```python
from build123d import *

# Parameters (mm, degrees)
BOSS_EXTRUDE1_DEPTH = 17
SKETCH2_R           = 3.9
CUT_EXTRUDE1_DEPTH  = 7.9
CUT_EXTRUDE2_START  = -7.9
SKETCH3_R           = 3.9
CUT_EXTRUDE2_DEPTH  = 7.9
SKETCH4_R           = 2.7
CUT_EXTRUDE3_DEPTH  = 1.2
SHELL1_DEPTH        = 15.8
SKETCH8_R           = 0.5
CUT_EXTRUDE4_DEPTH  = 17


# Read off the part's stored shape, not the designer's step: Shell1
with BuildPart() as part:
    # Sketch1 → Boss-Extrude1 (new body)
    with BuildSketch(Plane(origin=(0, 0, 0), x_dir=(1, 0, 0), z_dir=(0, 1, 0))):
        with BuildLine():
            Line((-9.1, 2.7), (-9.1, -2.7))
            add(Edge.make_bspline(
                [(-9.1, -2.7), (0, -7.5), (9.1, -2.7)],
                knots=[0, 0, 0, 1, 1, 1], degree=2))
            Line((9.1, -2.7), (9.1, 2.7))
            add(Edge.make_bspline(
                [(-9.1, 2.7), (0, 7.5), (9.1, 2.7)],
                knots=[0, 0, 0, 1, 1, 1], degree=2))
        make_face()
    extrude(amount=BOSS_EXTRUDE1_DEPTH)

    # Sketch2 → Cut-Extrude1 (cut)
    with BuildSketch(Plane(origin=(0, 17, 0), x_dir=(1, 0, 0), z_dir=(0, 1, 0))):
        with Locations(Location((0, 0, 0), (0, 0, 270))):
            Circle(SKETCH2_R)
    extrude(amount=-CUT_EXTRUDE1_DEPTH, mode=Mode.SUBTRACT)

    # Sketch3 → Cut-Extrude2 (cut)
    with BuildSketch(Plane(origin=(0, 0, 0), x_dir=(-1, 0, 0), z_dir=(0, -1, 0)).offset(CUT_EXTRUDE2_START)):
        with Locations(Location((0, 0, 0), (0, 0, 270))):
            Circle(SKETCH3_R)
    extrude(amount=CUT_EXTRUDE2_DEPTH, mode=Mode.SUBTRACT)

    # Sketch4 → Cut-Extrude3 (cut)
    with BuildSketch(Plane.XZ.offset(-7.9)):
        with Locations(Location((0, 0, 0), (0, 0, 270))):
            Circle(SKETCH4_R)
    extrude(amount=-CUT_EXTRUDE3_DEPTH, mode=Mode.SUBTRACT)

    # Shell1 outline → Shell1 (cut)
    with BuildSketch(Plane(origin=(0, 0, 0), x_dir=(1, 0, 0), z_dir=(0, 1, 0))):
        with BuildLine():
            Line((-7.899999781, 1.963775482), (-7.899999781, -1.963775482))
            add(Edge.make_bspline(
                [(-7.899999781, -1.963775482), (-7.481101996, -2.168383254), (-7.062952664, -2.360723495), (-6.645550136, -2.540844903), (-6.228886411, -2.708799004), (-5.812947019, -2.864639229), (-5.397710236, -3.008420202), (-4.983146308, -3.140196716), (-4.569217021, -3.260022384), (-4.155875768, -3.367948145), (-3.7430681, -3.46402079)],
                knots=[0.036996465, 0.036996465, 0.036996465, 0.036996465, 0.036996465, 0.036996465, 0.036996465, 0.036996465, 0.036996465, 0.036996465, 0.036996465, 0.279391491, 0.279391491, 0.279391491, 0.279391491, 0.279391491, 0.279391491, 0.279391491, 0.279391491, 0.279391491, 0.279391491, 0.279391491], degree=10))
            ThreePointArc((-3.7430681, -3.46402079), (-5.1, 0), (-3.74306828, 3.464020764))
            add(Edge.make_bspline(
                [(-3.74306828, 3.464020764), (-4.155875768, 3.367948145), (-4.569217021, 3.260022384), (-4.983146308, 3.140196716), (-5.397710236, 3.008420202), (-5.812947019, 2.864639229), (-6.228886411, 2.708799004), (-6.645550136, 2.540844903), (-7.062952664, 2.360723495), (-7.481101996, 2.168383254), (-7.899999781, 1.963775482)],
                knots=[0.720608509, 0.720608509, 0.720608509, 0.720608509, 0.720608509, 0.720608509, 0.720608509, 0.720608509, 0.720608509, 0.720608509, 0.720608509, 0.963003535, 0.963003535, 0.963003535, 0.963003535, 0.963003535, 0.963003535, 0.963003535, 0.963003535, 0.963003535, 0.963003535, 0.963003535], degree=10))
        make_face()
        with BuildLine():
            ThreePointArc((3.74306828, 3.464020764), (5.1, 0), (3.74306828, -3.464020764))
            add(Edge.make_bspline(
                [(3.74306828, -3.464020764), (4.155875768, -3.367948145), (4.569217021, -3.260022384), (4.983146308, -3.140196716), (5.397710236, -3.008420202), (5.812947019, -2.864639229), (6.228886411, -2.708799004), (6.645550136, -2.540844903), (7.062952664, -2.360723495), (7.481101996, -2.168383254), (7.899999781, -1.963775482)],
                knots=[0.720608509, 0.720608509, 0.720608509, 0.720608509, 0.720608509, 0.720608509, 0.720608509, 0.720608509, 0.720608509, 0.720608509, 0.720608509, 0.963003535, 0.963003535, 0.963003535, 0.963003535, 0.963003535, 0.963003535, 0.963003535, 0.963003535, 0.963003535, 0.963003535, 0.963003535], degree=10))
            Line((7.899999781, -1.963775482), (7.899999781, 1.963775482))
            add(Edge.make_bspline(
                [(7.899999781, 1.963775482), (7.481101996, 2.168383254), (7.062952664, 2.360723495), (6.645550136, 2.540844903), (6.228886411, 2.708799004), (5.812947019, 2.864639229), (5.397710236, 3.008420202), (4.983146308, 3.140196716), (4.569217021, 3.260022384), (4.155875768, 3.367948145), (3.74306828, 3.464020764)],
                knots=[0.036996465, 0.036996465, 0.036996465, 0.036996465, 0.036996465, 0.036996465, 0.036996465, 0.036996465, 0.036996465, 0.036996465, 0.036996465, 0.279391491, 0.279391491, 0.279391491, 0.279391491, 0.279391491, 0.279391491, 0.279391491, 0.279391491, 0.279391491, 0.279391491, 0.279391491], degree=10))
        make_face()
    extrude(amount=SHELL1_DEPTH, mode=Mode.SUBTRACT)

    # Sketch8 → Cut-Extrude4 (cut)
    with BuildSketch(Plane.XZ):
        with Locations((-3.9, 4.659183673)):
            Circle(SKETCH8_R)
        with Locations((-3.9, -4.659183673)):
            Circle(SKETCH8_R)
    cut_extrude4 = extrude(amount=-CUT_EXTRUDE4_DEPTH, mode=Mode.SUBTRACT)

    # Mirror1: Cut-Extrude4 across plane
    add(cut_extrude4.mirror(Plane(origin=(0, 0, 0), x_dir=(0, 0, 1), z_dir=(1, 0, 0))), mode=Mode.SUBTRACT)


solid = part.part
```
CAD build for the part. Positions are in the model's coordinates, mm. A direction names the side the tool comes from. Round coordinates to 2 decimals unless told otherwise and drop trailing zeros. Order: outer loops, then holes, each group sorted by start corner. A loop starts at its lowest first (then second) coordinate and runs counter-clockwise, first axis right, second up. Notation, with made-up numbers: (-34.5, 45) - (-11.5, 45) arc R33 cw to (-11.5, 84) - close; hole circle Ø9 at (-5, 55.25). An arc over 180 degrees is marked (long way). Answer in a Markdown table with one row per item. Add a question column.
(1) 3-axis set-ups, long thin cutter, end or side, ignore diameter. For faces 1 (the face through (-2.373, 13.105, -3.095)), 2 (the face through (-7.9, 8, 0)), 3 (the face through (-9.1, 8, 0)): which of +Z, -Z, +X, -X, +Y, -Y reach the whole face in a straight line?
(2) Probe L1, parallel to X at y = 4.5, z = 2.5; L2, parallel to Y at x = 7.5, z = 2; L3, parallel to X at y = 13, z = 1.25. List the from-to ranges inside material, lowest first. Write a range as [from, to].
(3) Band-saw the part on B-B on y = 8.75. Count the separate pieces of the cut face and the enclosed holes in it, and give its area (3 significant figures).
(4) Band-saw the part on A-A on z = 0. List the corners of the cut face in (x, y).
(5) Band-saw the part on C-C on z = -1.5. List the corners of the cut face in (x, y) (3 decimals), and give its area (3 significant figures).
(6) Drop flat-ended pins along their axis: pin 1 Ø4.5 at (x, z) = (0, 0) entering from +Y; pin 2 Ø6 at (x, z) = (0, 0) entering from -Y; pin 3 Ø3 at (x, y) = (-4.5, 14) entering from +Z. Give the stop position or say it passes through.
Data:
| question | item | result |
|---|---|---|
| 1 | face 1 | +Y |
| 1 | face 2 | -Y |
| 1 | face 3 | +Z, -Z, -X, +Y, -Y |
| 2 | L1 | x = [-9.1, -6.71], [-4.45, -2.99], [2.99, 4.45], [6.71, 9.1] |
| 2 | L2 | y = [15.8, 17] |
| 2 | L3 | x = [-9.1, -7.9], [-4.94, -3.69], [3.69, 4.94], [7.9, 9.1] |
| 3 | separate pieces | 1 |
| 3 | enclosed holes | 3 |
| 3 | area | 98.4 mm^2 |
| 4 | outline | (-9.1, 0) - (-7.9, 0) - (-7.9, 15.8) - (-5.1, 15.8) - (-5.1, 0) - (-3.9, 0) - (-3.9, 7.9) - (-2.7, 7.9) - (-2.7, 9.1) - (-3.9, 9.1) - (-3.9, 17) - (-9.1, 17) - close; (2.7, 7.9) - (3.9, 7.9) - (3.9, 0) - (5.1, 0) - (5.1, 15.8) - (7.9, 15.8) - (7.9, 0) - (9.1, 0) - (9.1, 17) - (3.9, 17) - (3.9, 9.1) - (2.7, 9.1) - close |
| 5 | outline | (-9.1, 0) - (-7.9, 0) - (-7.9, 15.8) - (-4.874, 15.8) - (-4.874, 0) - (-3.6, 0) - (-3.6, 7.9) - (-2.245, 7.9) - (-2.245, 9.1) - (-3.6, 9.1) - (-3.6, 17) - (-9.1, 17) - close; (2.245, 7.9) - (3.6, 7.9) - (3.6, 0) - (4.874, 0) - (4.874, 15.8) - (7.9, 15.8) - (7.9, 0) - (9.1, 0) - (9.1, 17) - (3.6, 17) - (3.6, 9.1) - (2.245, 9.1) - close |
| 5 | area | 94.6 mm^2 |
| 6 | pin 1 | passes through |
| 6 | pin 2 | stops at y = 7.9 |
| 6 | pin 3 | stops at z = 4.84 |
